The drawing under review shows one solid part. Ordinate dimensions are in mm from its lowest x, y, z. A direction names the side the tool comes from. Give positions to 0.01 mm unless a question says otherwise; leave off trailing zeros. Write each loop counter-clockwise with the first axis right and the second up, starting at its lowest first coordinate (ties: lowest second). Pieces come first, ordered by that corner, then holes. Notation, with made-up numbers: (-3, 26.5) - (32, 26.5) arc R29 cw to (32, 46.5) - close; hole circle Ø7 at (-5, 35.5). An arc over 180 degrees is marked (long way). Write item = value, one per line.
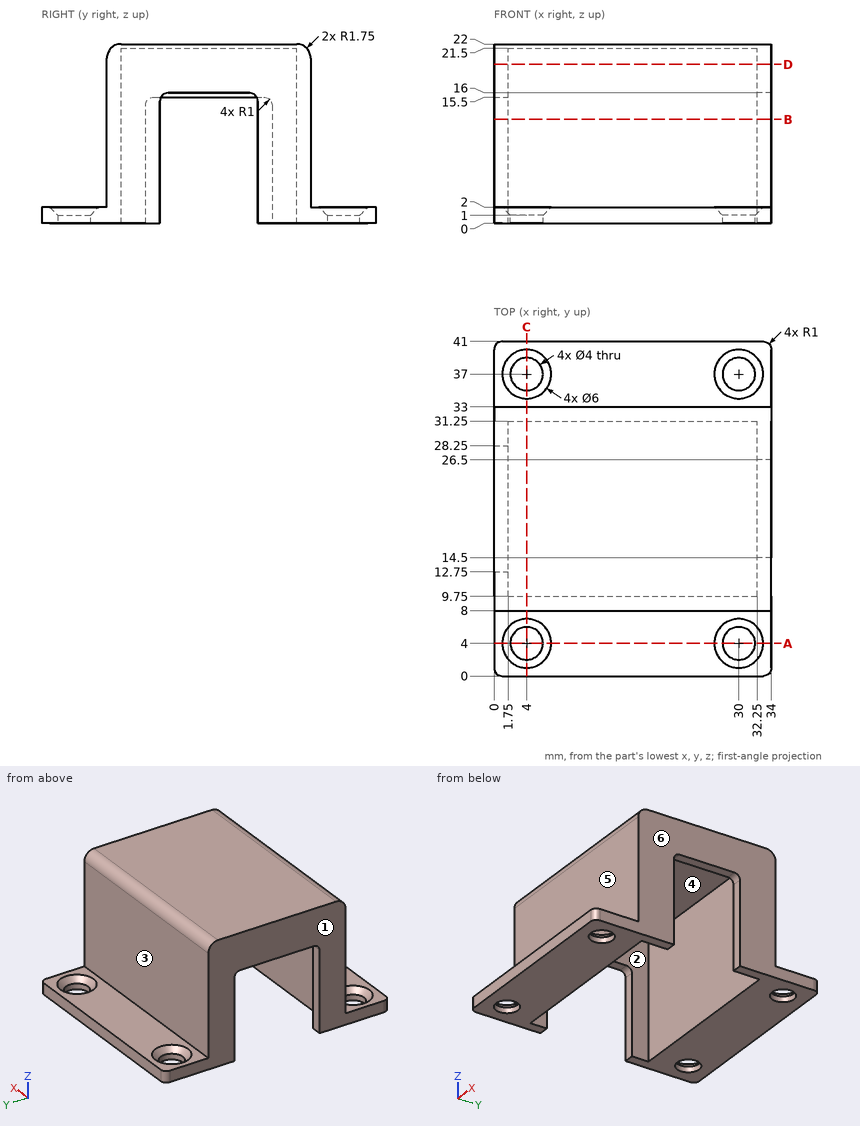
1. Draft analysis for pull direction X (two halves, no side actions). For the marked faces 4, 5 and 6, state which applies: +X half, -X half, draft (parallel to the pull), parting line (faces both ways), or undercut.
Findings below:
face_4 = undercut
face_5 = draft
face_6 = +X half
2. Take a section at D-D on z = 19.5. Give the boundary of the cut face in (x, y).
Findings below:
outline = (0, 8) - (34, 8) - (34, 33) - (0, 33) - close; hole (1.75, 9.75) - (32.25, 9.75) - (32.25, 31.25) - (1.75, 31.25) - close
3. Take a section at B-B on z = 12.75. Give the boundary of the cut face in (x, y).
Findings below:
outline = (0, 8) - (34, 8) - (34, 14.5) - (32.25, 14.5) - (32.25, 9.75) - (1.75, 9.75) - (1.75, 12.75) - (0, 12.75) - close; (0, 28.25) - (1.75, 28.25) - (1.75, 31.25) - (32.25, 31.25) - (32.25, 26.5) - (34, 26.5) - (34, 33) - (0, 33) - close
4. Machinability: for the marked faces 1, 2 and 3, which of the approach directions +Z, -Z, +X, -X, +Y, -Y give a long, thin tool a straight path to every point of the face, cutting with its end or side? Answer none if there is none.
Findings below:
face_1 = +Z, -Z, -X, +Y, -Y
face_2 = -Z
face_3 = +Z, +X, -X, +Y
5. Take a section at A-A on y = 4. Give the boundary of the cut face in (x, z).
Findings below:
outline = (0, 0) - (2, 0) - (2, 1) - (1, 2) - (0, 2) - close; (6, 0) - (28, 0) - (28, 1) - (27, 2) - (7, 2) - (6, 1) - close; (32, 0) - (34, 0) - (34, 2) - (33, 2) - (32, 1) - close
6. Insertion check: P1, Ø6.5, axis at x = 30, y = 37, coming from the +Z side; P2, Ø10, axis at x = 20.5, z = 11.5, coming from the +Y side; P3, Ø2, axis at y = 27, z = 9.5, coming from the -X side; P4, Ø2.5, axis at x = 30, y = 4, coming from the +Z side. Each pin has a flat end and moves straight along its axis. Give the tip position at first contact, or say it passes through.
Findings below:
P1 = 2
P2 = 33
P3 = 32.25
P4 = through
7. For line 1 (X direction, y = 37, z = 0.35); line 2 (Y direction, x = 29.5, z = 4); line 3 (X direction, y = 13, z = 19.5), list the stretches that pass through material, from the lowest coordinate up. Write a range as from..to.
Findings below:
line_1 = 0..2, 6..28, 32..34
line_2 = 8..9.75, 31.25..33
line_3 = 0..1.75, 32.25..34
8. Take a section at C-C on x = 4. Give the boundary of the cut face in (y, z).
Findings below:
outline = (0, 0) - (2, 0) - (2, 1) - (1, 2) - (0, 2) - close; (6, 0) - (9.75, 0) - (9.75, 21.5) - (31.25, 21.5) - (31.25, 0) - (35, 0) - (35, 1) - (34, 2) - (33, 2) - (33, 20.25) arc R1.75 ccw to (31.25, 22) - (9.75, 22) arc R1.75 ccw to (8, 20.25) - (8, 2) - (7, 2) - (6, 1) - close; (39, 0) - (41, 0) - (41, 2) - (40, 2) - (39, 1) - close
